Verification items for the finished model (mm, model axes). Face numbers are marked on the shaded views. A direction names the side the tool comes from. Round coordinates to 2 decimals unless told otherwise and drop trailing zeros. Write each loop counter-clockwise with the first axis right and the second up, starting at its lowest first coordinate (ties: lowest second). Pieces come first, ordered by that corner, then holes. Notation, with made-up numbers: (-12, -24) - (0, -24) arc R24 ccw to (0, -12) - close; hole circle Ø10 at (74.25, 6.5). An arc over 180 degrees is marked (long way). Write each question's results on one line, items separated by ' | '.
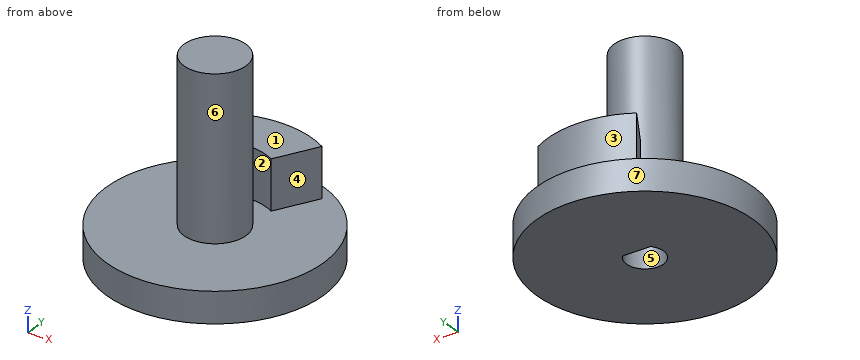
```python
from build123d import *

# Parameters (mm, degrees)
SKETCH1_R           = 17.5
BOSS_EXTRUDE1_DEPTH = 2.5
BOSS_EXTRUDE2_DEPTH = 8
SKETCH3_R           = 5
BOSS_EXTRUDE3_DEPTH = 26
CUT_EXTRUDE1_DEPTH  = 10


with BuildPart() as part:
    # Sketch1 → Boss-Extrude1 (new, symmetric)
    with BuildSketch(Plane.XY):
        Circle(SKETCH1_R)
    extrude(amount=BOSS_EXTRUDE1_DEPTH, both=True)

    # Sketch2 → Boss-Extrude2 (add)
    with BuildSketch(Plane.XY.offset(2.5)):
        with BuildLine():
            Line((7.875, 13.63990011), (4.125, 7.144709581))
            ThreePointArc((4.125, 7.144709581), (0, 8.25), (-4.125, 7.144709581))
            Line((-4.125, 7.144709581), (-7.875, 13.63990011))
            ThreePointArc((-7.875, 13.63990011), (0, 15.75), (7.875, 13.63990011))
        make_face()
    extrude(amount=BOSS_EXTRUDE2_DEPTH)

    # Sketch3 → Boss-Extrude3 (add)
    with BuildSketch(Plane.XY.offset(2.5)):
        with Locations(Location((0, 0, 0), (0, 0, 180))):
            Circle(SKETCH3_R)
    extrude(amount=BOSS_EXTRUDE3_DEPTH)

    # Sketch4 → Cut-Extrude1 (cut)
    with BuildSketch(Plane(origin=(0, 0, -2.5), x_dir=(-1, 0, 0), z_dir=(0, 0, -1))):
        with BuildLine():
            Line((-2.236067977, 2), (2.236067977, 2))
            ThreePointArc((2.236067977, 2), (0, -3), (-2.236067977, 2))
        make_face()
    extrude(amount=-CUT_EXTRUDE1_DEPTH, mode=Mode.SUBTRACT)


solid = part.part
```
(1) Section check D-D (z = 8). Record the cut outline in (x, y) (3 decimals).
Answer:
outline: (-7.875, 13.64) - (-4.125, 7.145) arc R8.25 cw to (4.125, 7.145) - (7.875, 13.64) arc R15.75 ccw to start; circle Ø10 at (0, 0)
(2) Go/stop test with flat-tipped pins: pin 1 Ø4 at (x, z) = (3, 14) entering from +Y; pin 2 Ø1.5 at (x, y) = (-0.5, -1.5) entering from -Z; pin 3 Ø4 at (y, z) = (13.5, 4) entering from +X. Record where each tip stops, or that it passes through.
Answer:
pin 1: y = 4.9 | pin 2: z = 7.5 | pin 3: x = 12.57
(3) Thickness scan on L1, parallel to Z at x = 0, y = 1.5; L2, parallel to Z at x = -3.5, y = 12; L3, parallel to Y at x = -0.5, z = 4. Record the ranges inside material, lowest first.
Answer:
L1: 7.5 to 28.5 | L2: -2.5 to 10.5 | L3: -4.97 to -2.96, 2 to 4.97, 8.23 to 15.74
(4) Set-up check for the marked faces 5, 6 and 7: record each of +Z, -Z, +X, -X, +Y, -Y from which the full face is reachable in a straight line by a thin tool's end or side.
Answer:
face 5: -Z | face 6: +Z | face 7: +Z, -Z
(5) Section check A-A (z = 3). Record the cut outline in (x, y) (3 decimals).
Answer:
outline: (-7.875, 13.64) - (-4.125, 7.145) arc R8.25 cw to (4.125, 7.145) - (7.875, 13.64) arc R15.75 ccw to start; circle Ø10 at (0, 0); hole (-2.236, 2) arc R3 ccw (long way) to (2.236, 2) - close
(6) Section check C-C (x = 0). Record the cut outline in (y, z).
Answer:
outline: (-17.5, -2.5) - (-3, -2.5) - (-3, 7.5) - (2, 7.5) - (2, -2.5) - (17.5, -2.5) - (17.5, 2.5) - (15.75, 2.5) - (15.75, 10.5) - (8.25, 10.5) - (8.25, 2.5) - (5, 2.5) - (5, 28.5) - (-5, 28.5) - (-5, 2.5) - (-17.5, 2.5) - close
(7) Section check B-B (y = 0). Record the cut outline in (x, z), plus the area to 3 significant figures.
Answer:
outline: (-17.5, -2.5) - (-3, -2.5) - (-3, 7.5) - (3, 7.5) - (3, -2.5) - (17.5, -2.5) - (17.5, 2.5) - (5, 2.5) - (5, 28.5) - (-5, 28.5) - (-5, 2.5) - (-17.5, 2.5) - close | area: 375 mm2
(8) Mould release check, pull along Y, two halves, no side actions. Record for the marked faces 1, 2, 3 and 4: released by +Y, released by -Y, zero draft, split by the parting line, or undercut.
Answer:
face 1: zero draft | face 2: undercut | face 3: released by +Y | face 4: undercut
